Build history of the part. All positions in model axes, mm. Round coordinates to 2 decimals unless told otherwise and drop trailing zeros. Order: outer loops, then holes, each group sorted by start corner. A loop starts at its lowest first (then second) coordinate and runs counter-clockwise, first axis right, second up. Notation, with made-up numbers: (-29, 29.5) -> (-19, 29.5) arc R29 ccw to (-19, 56.5) -> close; hole circle Ø8 at (-30.75, 41.25). An arc over 180 degrees is marked (long way). Use a Markdown table: item, result. Add a question column.
Item 1: Probe L1, parallel to Y at x = 12.5, z = 5; L2, parallel to Y at x = 9, z = 4.5; L3, parallel to X at y = 26, z = 2.75. List the from-to ranges inside material, lowest first.
Item 2: Pin check, flat tips, straight feed: pin 1 (1.5 mm diameter, centred on x = 18, z = 2, fed in from -Y); pin 2 (5 mm diameter, centred on x = 11.5, z = 7, fed in from -Y); pin 3 (5 mm diameter, centred on x = 5.5, z = 3.5, fed in from +Y). Stop position of each tip, or through.
Item 3: Two-plate mould, pull along Y, no slides. Class faces 1 (the face through (31.1, -0.68, 0.12)), 2 (the face through (0.444, -27, 5)), 3 (the face through (22.35, 0.49, 0.63)): released by +Y, released by -Y, zero draft, split by the parting line, or undercut.
Item 4: Slice it at A-A, the plane y = 0. Give the cut face in (x, z) (3 decimals), plus the area to 3 significant figures.
from build123d import *

# Parameters (mm, degrees)
F1_DEPTH = 9.525
F2_SIZE  = 0.762


with BuildPart() as f1:
    # F0 (on Top) → F1 (new body)
    with BuildSketch(Plane.XY):
        with BuildLine():
            ThreePointArc((0.4445, 22.220555), (22.225, 0), (0.4445, -22.220555))
            Line((0.4445, -22.220555), (0.4445, -31.746888))
            ThreePointArc((0.4445, -31.746888), (31.75, 0), (0.4445, 31.746888))
            Line((0.4445, 31.746888), (0.4445, 22.220555))
        make_face()
    extrude(amount=F1_DEPTH)

    # F2
    f2_edges = [f1.edges().sort_by_distance(p)[0] for p in [
        (31.75, 0, 9.525),
        (31.75, 0, 0),
        (22.225, 0, 9.525),
        (22.225, 0, 0),
    ]]
    chamfer(f2_edges, length=F2_SIZE)


solid = f1.part
Check sheet entries:
| question | item | result |
|---|---|---|
| 1 | L1 | -29.19 to -18.38, 18.38 to 29.19 |
| 1 | L2 | -30.45 to -20.32, 20.32 to 30.45 |
| 1 | L3 | 0.44 to 18.22 |
| 2 | pin 1 | y = -26.66 |
| 2 | pin 2 | y = -30.45 |
| 2 | pin 3 | y = 31.61 |
| 3 | face 1 | split by the parting line |
| 3 | face 2 | zero draft |
| 3 | face 3 | undercut |
| 4 | outline | (22.225, 0.762) -> (22.987, 0) -> (30.988, 0) -> (31.75, 0.762) -> (31.75, 8.763) -> (30.988, 9.525) -> (22.987, 9.525) -> (22.225, 8.763) -> close |
| 4 | area | 89.6 mm2 |
